Input: dimensioned drawing with shaded views. Units: mm. Origin: part minimum x, y, z. Give positions to 0.01 mm unless a question says otherwise; leave off trailing zeros. Loops run counter-clockwise (first coordinate to the right, second up) from the corner with the lowest first, then second, coordinate; pieces in that order, holes last. Notation, with made-up numbers: M -25,4.5 L 16,4.5 A32 cw 16,31.5 Z; hole C 6,-36 d9. An arc over 180 degrees is marked long. Use CSV: the item, a comma, the result in double quotes. Start each with the question number.
Q1. Material intervals for line 1 along Y through (x, z) = (20, 9.5) (1 decimal); line 2 along Y through (x, z) = (40, 7) (1 decimal); line 3 along X through (y, z) = (45.5, 8.5) (1 decimal), sorted ascending.
Q2. Pin query (flat end, axial travel): pin 1 (6 mm diameter, centred on x = 22.5, z = 3.5, fed in from -Y) (1 decimal); pin 2 (1 mm diameter, centred on x = 43, z = 2, fed in from +Y); pin 3 (1.5 mm diameter, centred on x = 8.5, z = 15.5, fed in from +Y). Return the tip coordinate at first contact, or that it passes through.
Q3. Section D-D, the plane x = 20. Output: boundary loops of the cut face in (y, z) (1 decimal), plus the area to 3 significant figures.
Q4. Section C-C, the plane x = 41.5. Output: boundary loops of the cut face in (y, z) (1 decimal), plus the area to 3 significant figures.
Q5. Section A-A, the plane x = 33. Output: boundary loops of the cut face in (y, z), plus the area to 3 significant figures.
Q6. Section B-B, the plane z = 14. Output: boundary loops of the cut face in (x, y).
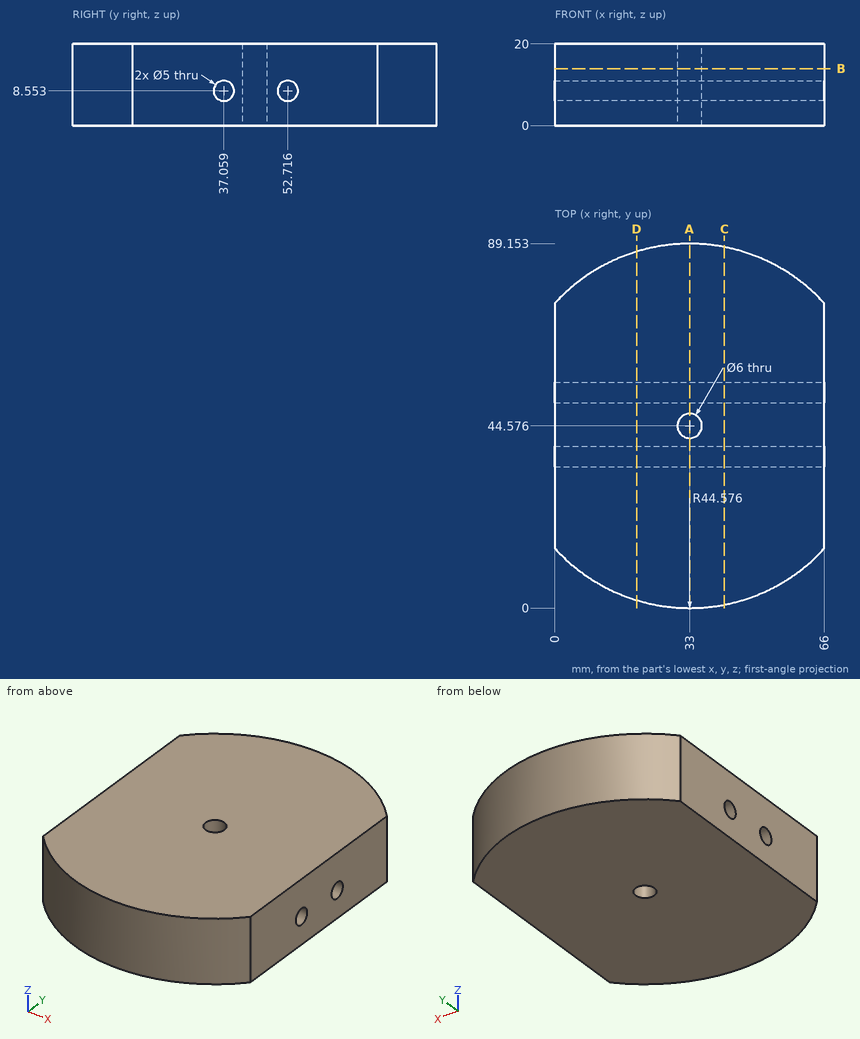
A:
1,line 1,"1.9 to 34.7, 39.4 to 50.4, 55 to 87.2"
1,line 2,"0.6 to 35.1, 39 to 50.8, 54.7 to 88.6"
1,line 3,"0 to 30.1, 35.9 to 66"
2,pin 1,"y = 0.6"
2,pin 2,"y = 88.13"
2,pin 3,"y = 82.3"
3,outline,"M 1.9,0 L 87.2,0 L 87.2,20 L 1.9,20 Z; hole C 37.1,8.6 d5; hole C 52.7,8.6 d5"
3,area,"1,670 mm^2"
4,outline,"M 0.8,0 L 88.3,0 L 88.3,20 L 0.8,20 Z; hole C 37.1,8.6 d5; hole C 52.7,8.6 d5"
4,area,"1,710 mm^2"
5,outline,"M 0,0 L 41.58,0 L 41.58,20 L 0,20 Z; M 47.58,0 L 89.15,0 L 89.15,20 L 47.58,20 Z; hole C 37.06,8.55 d5; hole C 52.72,8.55 d5"
5,area,"1,620 mm^2"
6,outline,"M 0,14.61 A44.58 ccw 66,14.61 L 66,74.54 A44.58 ccw 0,74.54 Z; hole C 33,44.58 d6"
